```python
from build123d import *

# Parameters (mm, degrees)
SKETCH1_W           = 410
SKETCH1_H           = 150
BOSS_EXTRUDE1_DEPTH = 3
CUT_EXTRUDE1_DEPTH  = 3
SKETCH3_R           = 2
CUT_EXTRUDE2_DEPTH  = 3
SKETCH4_R           = 2
SKETCH4_R_2         = 17.5
CUT_EXTRUDE3_DEPTH  = 10
SKETCH5_W           = 35
SKETCH5_H           = 24
CUT_EXTRUDE4_DEPTH  = 10


with BuildPart() as part:
    # Sketch1 → Boss-Extrude1 (new body)
    with BuildSketch(Plane(origin=(0, 0, 0), x_dir=(0, 0, -1), z_dir=(1, 0, 0))):
        with Locations((205, 75)):
            Rectangle(SKETCH1_W, SKETCH1_H)
    extrude(amount=BOSS_EXTRUDE1_DEPTH)

    # Sketch2 → Cut-Extrude1 (cut)
    with BuildSketch(Plane(origin=(3, 0, 0), x_dir=(0, 0, -1), z_dir=(1, 0, 0))):
        Polygon((145, 150), (0, 75), (0, 150), align=None)
        Polygon((265, 150), (410, 75), (410, 150), align=None)
    extrude(amount=-CUT_EXTRUDE1_DEPTH, mode=Mode.SUBTRACT)

    # Sketch3 → Cut-Extrude2 (cut)
    with BuildSketch(Plane(origin=(3, 0, 0), x_dir=(0, 0, -1), z_dir=(1, 0, 0))):
        with Locations((45, 50)):
            Circle(SKETCH3_R)
        with Locations((125, 50)):
            Circle(SKETCH3_R)
        with Locations((205, 50)):
            Circle(SKETCH3_R)
        with Locations((285, 50)):
            Circle(SKETCH3_R)
        with Locations((365, 50)):
            Circle(SKETCH3_R)
    extrude(amount=-CUT_EXTRUDE2_DEPTH, mode=Mode.SUBTRACT)

    # Sketch4 → Cut-Extrude3 (cut)
    with BuildSketch(Plane(origin=(3, 0, 0), x_dir=(0, 0, -1), z_dir=(1, 0, 0))):
        with Locations((176, 126)):
            Circle(SKETCH4_R)
        with Locations((176.845, 119.051188951)):
            Circle(SKETCH4_R)
        with Locations((205, 126)):
            Circle(SKETCH4_R_2)
        with Locations(Location((233.155, 119.051188951, 0), (0, 0, 180))):
            Circle(SKETCH4_R)
        with Locations(Location((234, 126, 0), (0, 0, 180))):
            Circle(SKETCH4_R)
    extrude(amount=-CUT_EXTRUDE3_DEPTH, mode=Mode.SUBTRACT)

    # Sketch5 → Cut-Extrude4 (cut)
    with BuildSketch(Plane(origin=(3, 0, 0), x_dir=(0, 0, -1), z_dir=(1, 0, 0))):
        with Locations((205, 138)):
            Rectangle(SKETCH5_W, SKETCH5_H)
    extrude(amount=-CUT_EXTRUDE4_DEPTH, mode=Mode.SUBTRACT)


solid = part.part
```
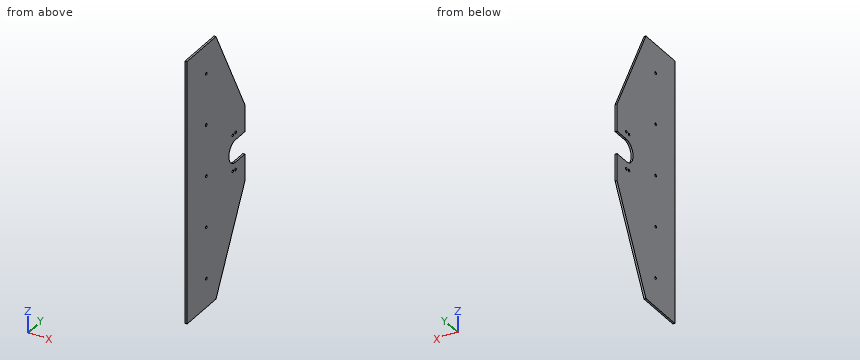
Here's how the part is built. I have some questions about the finished solid (model axes, mm). Round coordinates to 2 decimals unless told otherwise and drop trailing zeros. Order: outer loops, then holes, each group sorted by start corner. A loop starts at its lowest first (then second) coordinate and runs counter-clockwise, first axis right, second up. Notation, with made-up numbers: M 3.5,83 L 27.5,83 A30 cw 27.5,106 Z; hole C -24,-22.5 d10. An arc over 180 degrees is marked long. Use CSV: the item, a comma, the result in double quotes.
1) I want a section at A-A (x = 2.1). Count the separate pieces of the cut face and the enclosed holes in it, then the cut area to 3 significant figures.
Taken from the geometry:
separate pieces,"1"
enclosed holes,"9"
area,"49,200 mm^2"
2) I want a section at B-B (z = -308.5). List the corners of the cut face in (x, y) for me.
Taken from the geometry:
outline,"M 0,0 L 3,0 L 3,127.5 L 0,127.5 Z"
3) I need wall thicknesses on line 1 along Y through (x, z) = (2.15, -176); line 2 along Y through (x, z) = (2.1, -205); line 3 along Z through (x, y) = (2.8, 127). Which ranges of each line are inside material? Lowest first, please. Write a range as [from, to].
Taken from the geometry:
line 1,"[0, 117.24], [120.86, 124], [128, 150]"
line 2,"[0, 48], [52, 108.5]"
line 3,"[-309.47, -235.73], [-232.27, -222.5], [-187.5, -177.73], [-174.27, -100.53]"
4) I'm going to push flat-ended pins straight in: P1, Ø1.5, axis at x = 1, z = -211, coming from the +Y side; P2, Ø3.5, axis at y = 50, z = -125, coming from the -X side; P3, Ø1.5, axis at x = 1.5, y = 138, coming from the +Z side. Where does each tip first touch, or does it pass through?
Taken from the geometry:
P1,"y = 109.85"
P2,"through"
P3,"z = -120.35"
5) I want a section at C-C (y = 100). List the corners of the cut face in (x, z) for me, then the cut area to 3 significant figures.
Taken from the geometry:
outline,"M 0,-361.67 L 3,-361.67 L 3,-48.33 L 0,-48.33 Z"
area,"940 mm^2"
